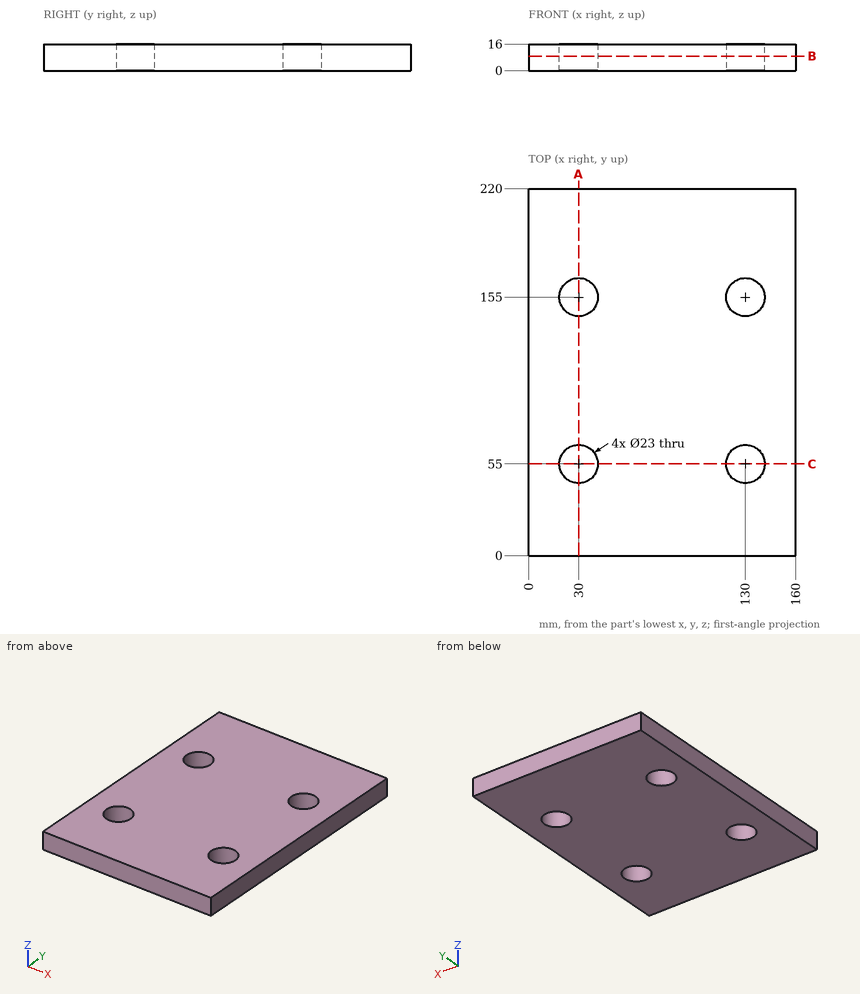
Geometry: see drawing. Coordinates: mm, zero at the bounding-box minimum. Coordinates: 2 decimals unless noted, no trailing zeros. Order: outer loops, then holes, each group sorted by start corner. A loop starts at its lowest first (then second) coordinate and runs counter-clockwise, first axis right, second up. Notation, with made-up numbers: M -10.75,-11.75 L 25.25,-11.75 A11 ccw 25.25,4.25 Z; hole C -24,-24.75 d7. An arc over 180 degrees is marked long. Answer as CSV lines item,"result".
1. Section A-A (x = 30). Return the cut outline in (y, z), then the cut area to 3 significant figures.
Reported:
outline,"M 0,0 L 43.5,0 L 43.5,16 L 0,16 Z; M 66.5,0 L 143.5,0 L 143.5,16 L 66.5,16 Z; M 166.5,0 L 220,0 L 220,16 L 166.5,16 Z"
area,"2,780 mm2"
2. Section B-B (z = 8.75). Return the cut outline in (x, y).
Reported:
outline,"M 0,0 L 160,0 L 160,220 L 0,220 Z; hole C 30,55 d23; hole C 30,155 d23; hole C 130,55 d23; hole C 130,155 d23"
3. Material intervals for line 1 (Y direction, x = 129.5, z = 5.75); line 2 (X direction, y = 48.5, z = 1.25); line 3 (Y direction, x = 140.5, z = 14.5), sorted ascending. Write a range as from..to.
Reported:
line 1,"0..43.51, 66.49..143.51, 166.49..220"
line 2,"0..20.51, 39.49..120.51, 139.49..160"
line 3,"0..50.31, 59.69..150.31, 159.69..220"
4. Section C-C (y = 55). Return the cut outline in (x, z), then the cut area to 3 significant figures.
Reported:
outline,"M 0,0 L 18.5,0 L 18.5,16 L 0,16 Z; M 41.5,0 L 118.5,0 L 118.5,16 L 41.5,16 Z; M 141.5,0 L 160,0 L 160,16 L 141.5,16 Z"
area,"1,820 mm2"
